```python
from build123d import *

# Parameters (mm, degrees)
SKETCH1_R               = 4
BOSS_EXTRUDE1_DEPTH     = 28.83
SKETCH2_R               = 5.475
CUT_EXTRUDE1_DEPTH      = 5
CUT_EXTRUDE1_DEPTH_BACK = 5
SKETCH3_R               = 2.5
BOSS_EXTRUDE2_DEPTH     = 1


with BuildPart() as part:
    # Sketch1 → Boss-Extrude1 (new body)
    with BuildSketch(Plane(origin=(0, 0, 0), x_dir=(1, 0, 0), z_dir=(0, 1, 0))):
        Circle(SKETCH1_R)
    extrude(amount=BOSS_EXTRUDE1_DEPTH)

    # Sketch2 → Cut-Extrude1 (cut, two sides)
    with BuildSketch(Plane.XY) as cut_extrude1_sk:
        with Locations((6.1, 14.415)):
            Circle(SKETCH2_R)
    extrude(amount=CUT_EXTRUDE1_DEPTH, mode=Mode.SUBTRACT)
    extrude(cut_extrude1_sk.sketch, amount=-CUT_EXTRUDE1_DEPTH_BACK, mode=Mode.SUBTRACT)

    # Sketch3 → Boss-Extrude2 (add)
    with BuildSketch(Plane.XZ):
        with Locations((0, 0.069764056)):
            Circle(SKETCH3_R)
    extrude(amount=BOSS_EXTRUDE2_DEPTH)


solid = part.part
```
Geometry: final body of the model. Coordinates: model frame, mm. A direction names the side the tool comes from. Coordinates: 2 decimals unless noted, no trailing zeros. Order: outer loops, then holes, each group sorted by start corner. A loop starts at its lowest first (then second) coordinate and runs counter-clockwise, first axis right, second up. Notation, with made-up numbers: (26, -40) - (43, -40) arc R16 ccw to (43, -22) - close; hole circle Ø5 at (-12.75, 2). An arc over 180 degrees is marked (long way). Write each question's results on one line, items separated by ' | '.
(1) Set-up query: faces 4 (the face through (2, 0, -2)), 5 (the face through (-4, 14, 0)). Return all of +Z, -Z, +X, -X, +Y, -Y with unobstructed straight access to the full face (end or side cutting, diameter ignored); none if empty.
Values found:
face 4: -Y | face 5: +Y, -Y
(2) Mould query, pull axis Y, two halves, no side actions, for faces 1 (the face through (0, -1, 0)), 2 (the face through (0.626, 14.505, -0.055)), 3 (the face through (2.385, -0.493, 0.821)). Classes: +Y half, -Y half, draft (parallel to the pull), parting line (faces both ways), or undercut.
Values found:
face 1: -Y half | face 2: undercut | face 3: draft
(3) Section query D-D, the plane x = -3. Return the cut outline in (y, z).
Values found:
outline: (0, -2.65) - (28.83, -2.65) - (28.83, 2.65) - (0, 2.65) - close
(4) First-contact query: pin 1 Ø3 at (x, y) = (2.5, 6.5) entering from -Z. Flat tip, straight axial feed; report the tip coordinate or a pass-through.
Values found:
pin 1: stops at z = -3.87
(5) Section query C-C, the plane y = 24. Return the cut outline in (x, z), plus the area to 3 significant figures.
Values found:
outline: circle Ø8 at (0, 0) | area: 50.3 mm²
(6) Section query A-A, the plane x = -0.75. Return the cut outline in (y, z), plus the area to 3 significant figures.
Values found:
outline: (-1, -2.32) - (0, -2.32) - (0, -3.93) - (28.83, -3.93) - (28.83, 3.93) - (0, 3.93) - (0, 2.45) - (-1, 2.45) - close | area: 231 mm²
(7) Section query B-B, the plane z = 2.25. Return the cut outline in (x, y) (3 decimals), plus the area to 3 significant figures.
Values found:
outline: (-3.307, 0) - (-1.223, 0) - (-1.223, -1) - (1.223, -1) - (1.223, 0) - (3.307, 0) - (3.307, 9.706) arc R5.475 cw to (3.307, 19.124) - (3.307, 28.83) - (-3.307, 28.83) - close | area: 175 mm²
(8) Line query: line 1 (Y direction, x = 2, z = 1.5); line 2 (Y direction, x = -2, z = -2.25); line 3 (Y direction, x = 2.5, z = -3). Output: solid intervals per line, ascending. Write a range as [from, to].
Values found:
line 1: y = [-1, 10.79], [18.04, 28.83] | line 2: y = [0, 28.83] | line 3: y = [0, 10.29], [18.54, 28.83]
